from build123d import *

# Parameters (mm, degrees)
SKETCH_1_W          = 48
SKETCH_1_H          = 58
EXTRUDE_1_DEPTH     = 16
CUT_EXTRUDE_1_DEPTH = 41.902322672


with BuildPart() as part:
    # 草图1 → 凸台-拉伸1 (new body)
    with BuildSketch(Plane.XY):
        Rectangle(SKETCH_1_W, SKETCH_1_H)
    extrude(amount=-EXTRUDE_1_DEPTH)

    # 草图2 → 切除-拉伸1 (cut, through all)
    with BuildSketch(Plane.XY):
        with BuildLine():
            Line((-14, 4.5), (14, 4.5))
            ThreePointArc((14, 4.5), (18.5, 0), (14, -4.5))
            Line((14, -4.5), (-14, -4.5))
            ThreePointArc((-14, -4.5), (-18.5, 0), (-14, 4.5))
        make_face()
    extrude(amount=-CUT_EXTRUDE_1_DEPTH, mode=Mode.SUBTRACT)


solid = part.part
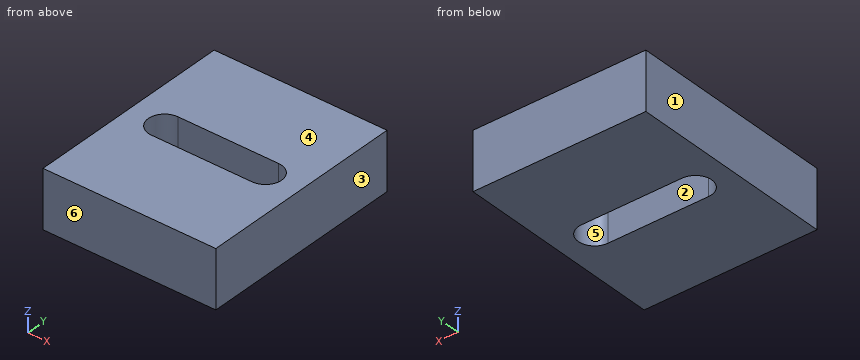
For this review, take the finished solid that the model builds, in its own axes (mm). Face numbers are marked on the shaded views. A direction names the side the tool comes from. Coordinates: 2 decimals unless noted, no trailing zeros. Write each loop counter-clockwise with the first axis right and the second up, starting at its lowest first coordinate (ties: lowest second). Pieces come first, ordered by that corner, then holes. Notation, with made-up numbers: (70.25, -14) -> (102.25, -14) arc R23 ccw to (102.25, -3) -> close; hole circle Ø1 at (18, -22.75). An arc over 180 degrees is marked (long way). Write each question's results on one line, items separated by ' | '. Start each with the question number.
1) The part is to be moulded in two halves that separate along X. For the marked faces 1, 2, 3 and 4, say which applies: +X half, -X half, draft (parallel to the pull), parting line (faces both ways), or undercut.
2) Insertion check: pin 1 (1 mm diameter, centred on x = -15.5, y = -23, fed in from +Z). The pin has a flat end and moves straight along its axis. Give the tip position at first contact, or say it passes through.
3) Wall thickness on L1, parallel to Y at x = -9.5, z = -0.25; L2, parallel to X at y = 1, z = -13; L3, parallel to Y at x = 17, z = -4: over which ranges is each line inside the solid? List them lowest first. Write a range as [from, to].
4) Consider section B-B (x = 8). Write out the cut boundary in (y, z), plus the area to 3 significant figures.
5) For the marked faces 5 and 6, list the 3-axis set-ups (+Z, -Z, +X, -X, +Y, -Y) from which the entire face can be reached by the end or side of a thin tool; tool diameter is ignored.
6) Consider section A-A (y = 0). Write out the cut boundary in (x, z), plus the area to 3 significant figures.
7) Consider section C-C (z = -5.25). Write out the cut boundary in (x, y).
Geometry says:
1) face 1: -X half | face 2: undercut | face 3: +X half | face 4: draft
2) pin 1: z = 0
3) L1: [-29, -4.5], [4.5, 29] | L2: [-24, -18.39], [18.39, 24] | L3: [-29, -3.35], [3.35, 29]
4) outline: (-29, -16) -> (-4.5, -16) -> (-4.5, 0) -> (-29, 0) -> close; (4.5, -16) -> (29, -16) -> (29, 0) -> (4.5, 0) -> close | area: 784 mm^2
5) face 5: +Z, -Z | face 6: +Z, -Z, +X, -X, -Y
6) outline: (-24, -16) -> (-18.5, -16) -> (-18.5, 0) -> (-24, 0) -> close; (18.5, -16) -> (24, -16) -> (24, 0) -> (18.5, 0) -> close | area: 176 mm^2
7) outline: (-24, -29) -> (24, -29) -> (24, 29) -> (-24, 29) -> close; hole (-14, -4.5) -> (14, -4.5) arc R4.5 ccw to (14, 4.5) -> (-14, 4.5) arc R4.5 ccw to start
